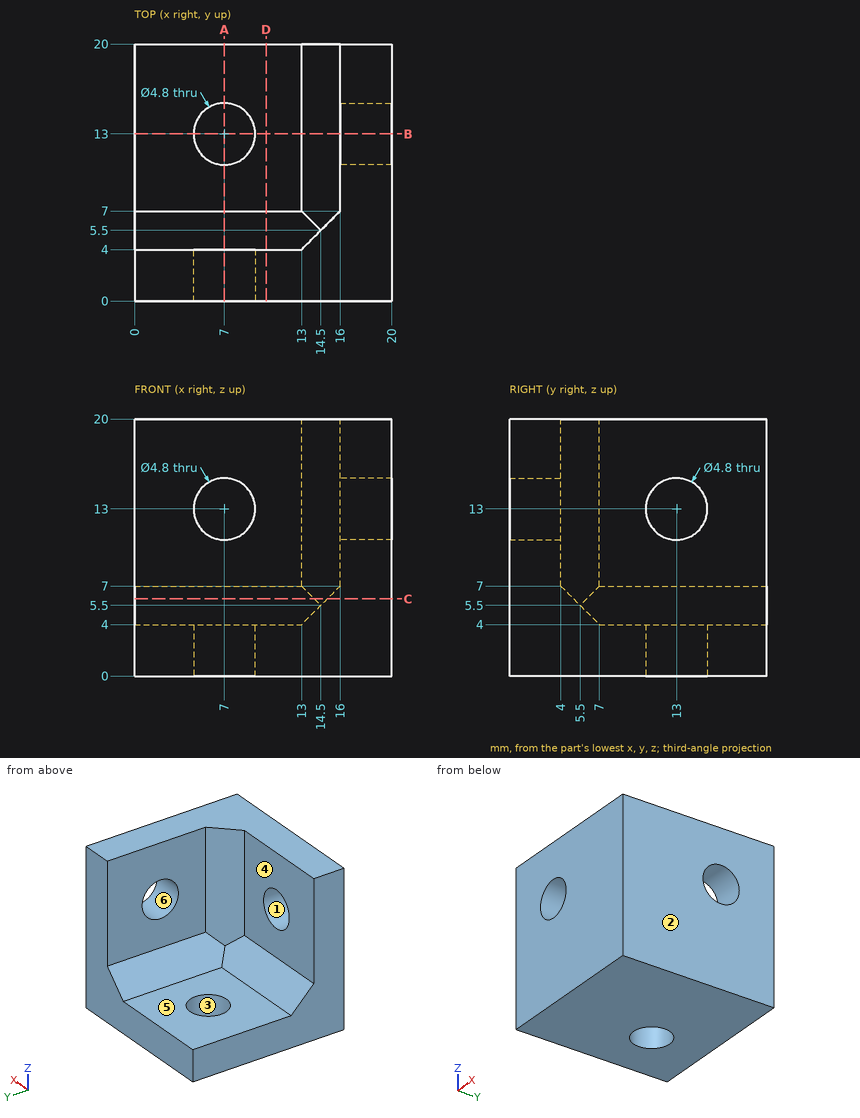
Part print with two shaded views. Sizes in mm from the minimum x, y, z corner. A direction names the side the tool comes from. Coordinates: 2 decimals unless noted, no trailing zeros. Order: outer loops, then holes, each group sorted by start corner. A loop starts at its lowest first (then second) coordinate and runs counter-clockwise, first axis right, second up.
(1) Saw through at C-C, the plane z = 6. Write the cut outline in (x, y).
Solution:
outline: (0, 0) - (20, 0) - (20, 20) - (15, 20) - (15, 6) - (14, 5) - (0, 5) - close
(2) Drill centre lines: L1, parallel to Z at x = 7, y = 1.7; L2, parallel to Y at x = 11.5, z = 19. Where is each one in solid material? Low to high.
Solution:
L1: z = 0 to 10.6, 15.4 to 20
L2: y = 0 to 4
(3) Saw through at D-D, the plane x = 10.25. Write the cut outline in (y, z).
Solution:
outline: (0, 0) - (20, 0) - (20, 4) - (7, 4) - (4, 7) - (4, 20) - (0, 20) - close
(4) Mould opens along X. For the marked faces 1, 2, 3 and 4 say: released by +X, released by -X, zero draft, split by the parting line, or undercut.
Solution:
face 1: undercut
face 2: released by +X
face 3: undercut
face 4: zero draft
(5) Saw through at A-A, the plane x = 7. Write the cut outline in (y, z).
Solution:
outline: (0, 0) - (10.6, 0) - (10.6, 4) - (7, 4) - (4, 7) - (4, 10.6) - (0, 10.6) - close; (0, 15.4) - (4, 15.4) - (4, 20) - (0, 20) - close; (15.4, 0) - (20, 0) - (20, 4) - (15.4, 4) - close
(6) Pin check, flat tips, straight feed: pin 1 Ø6.5 at (x, z) = (4.5, 11) entering from +Y; pin 2 Ø4 at (y, z) = (15, 12.5) entering from -X; pin 3 Ø4.5 at (x, y) = (7, 13) entering from +Z. Stop position of each tip, or through.
Solution:
pin 1: stops at y = 4
pin 2: stops at x = 16
pin 3: passes through
(7) Which spindle directions (+Z, -Z, +X, -X, +Y, -Y) get a long thin tool onto all of the face, cutting with end or side? Do the marked faces 5 and 6. Say none if no direction does.
Solution:
face 5: +Z, -X, +Y
face 6: +X, -X
(8) Saw through at B-B, the plane y = 13. Write the cut outline in (x, z).
Solution:
outline: (0, 0) - (4.6, 0) - (4.6, 4) - (0, 4) - close; (9.4, 0) - (20, 0) - (20, 10.6) - (16, 10.6) - (16, 7) - (13, 4) - (9.4, 4) - close; (16, 15.4) - (20, 15.4) - (20, 20) - (16, 20) - close
